For this review, use the dimensioned drawing (mm, ordinates from the lowest corner) and the shaded views. A direction names the side the tool comes from. Give positions to 0.01 mm unless a question says otherwise; leave off trailing zeros. Order: outer loops, then holes, each group sorted by start corner. A loop starts at its lowest first (then second) coordinate and runs counter-clockwise, first axis right, second up. Notation, with made-up numbers: (17.25, -14) - (71.25, -14) arc R24 ccw to (71.25, 24) - close; hole circle Ø9 at (23, 71). An arc over 180 degrees is marked (long way). One line per item, written item: value.
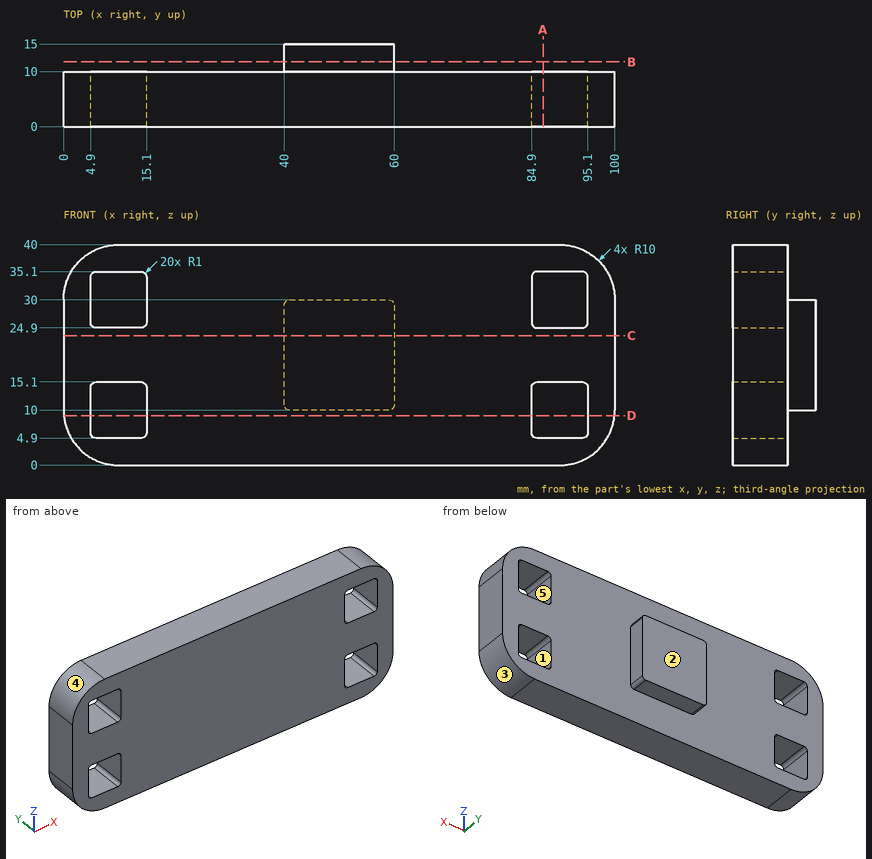
(1) Wall thickness on line 1 (Z direction, x = 10.5, y = 3); line 2 (X direction, y = 3.25, z = 29.5); line 3 (X direction, y = 3.5, z = 7): over which ranges is each line inside the solid? List them lowest first. Write a range as from..to.
Answers below:
line 1: z = 0..4.9, 15.1..24.9, 35.1..40
line 2: x = 0..4.9, 15.1..84.9, 95.1..100
line 3: x = 0.46..4.9, 15.1..84.9, 95.1..99.54
(2) Take a section at C-C (z = 23.5). Write out the cut boundary in (x, y).
Answers below:
outline: (0, 0) - (100, 0) - (100, 10) - (60, 10) - (60, 15) - (40, 15) - (40, 10) - (0, 10) - close
(3) Take a section at B-B (y = 11.75). Write out the cut boundary in (x, z), then the cut area to 3 significant figures.
Answers below:
outline: (40, 11) arc R1 ccw to (41, 10) - (59, 10) arc R1 ccw to (60, 11) - (60, 29) arc R1 ccw to (59, 30) - (41, 30) arc R1 ccw to (40, 29) - close
area: 399 mm^2
(4) Draft analysis for pull direction Z (two halves, no side actions). For the marked faces 1, 2 and 3, state which applies: pulls with the +Z half, pulls with the -Z half, needs draft (parallel to the pull), parting line crosses it, or undercut.
Answers below:
face 1: undercut
face 2: needs draft
face 3: pulls with the -Z half
(5) Take a section at A-A (x = 87). Write out the cut boundary in (y, z), then the cut area to 3 significant figures.
Answers below:
outline: (0, 0) - (10, 0) - (10, 4.9) - (0, 4.9) - close; (0, 15.1) - (10, 15.1) - (10, 24.9) - (0, 24.9) - close; (0, 35.1) - (10, 35.1) - (10, 40) - (0, 40) - close
area: 196 mm^2
(6) Machinability: for the marked faces 4 and 5, which of the approach directions +Z, -Z, +X, -X, +Y, -Y give a long, thin tool a straight path to every point of the face, cutting with its end or side? Answer none if there is none.
Answers below:
face 4: +Z, -X, +Y, -Y
face 5: +Y, -Y
(7) For P1, Ø9, axis at x = 91.5, y = 6.5, coming from the -Z side; P2, Ø2.5, axis at y = 3, z = 8, coming from the +X side; P3, Ø2.5, axis at y = 7, z = 8.5, coming from the -X side; P4, Ø1.5, axis at x = 13.5, z = 5, coming from the +Y side, all flat-tipped, find the tip position at first contact; note any pin that passes through.
Answers below:
P1: stops at z = 0
P2: stops at x = 99.97
P3: stops at x = 0
P4: stops at y = 10
(8) Take a section at D-D (z = 9). Write out the cut boundary in (x, y).
Answers below:
outline: (0.05, 0) - (4.9, 0) - (4.9, 10) - (0.05, 10) - close; (15.1, 0) - (84.9, 0) - (84.9, 10) - (15.1, 10) - close; (95.1, 0) - (99.95, 0) - (99.95, 10) - (95.1, 10) - close
